from build123d import *

# Parameters (mm, degrees)
SKETCH1_W           = 101.6
SKETCH1_H           = 53.34
BOSS_EXTRUDE1_DEPTH = 1.524
SKETCH2_W           = 19.05
SKETCH2_H           = 19.05
BOSS_EXTRUDE2_DEPTH = 1.016
SKETCH3_W           = 14.918140665
SKETCH3_H           = 9.726042688
BOSS_EXTRUDE3_DEPTH = 12.7
SKETCH4_W           = 24.926999196
SKETCH4_H           = 1.692574019
SKETCH4_W_2         = 22.820903589
SKETCH4_H_2         = 2.077249933
SKETCH4_W_3         = 16.079453185
SKETCH4_H_3         = 2.769666577
SKETCH4_W_4         = 2.00031475
SKETCH4_H_4         = 36.313406236
SKETCH4_W_5         = 30.004721254
SKETCH4_W_6         = 23.772971456
SKETCH4_H_5         = 2.615796212
BOSS_EXTRUDE4_DEPTH = 9.525


with BuildPart() as part:
    # Sketch1 → Boss-Extrude1 (new body)
    with BuildSketch(Plane(origin=(0, 0, 0), x_dir=(1, 0, 0), z_dir=(0, 1, 0))):
        Rectangle(SKETCH1_W, SKETCH1_H)
    extrude(amount=BOSS_EXTRUDE1_DEPTH)

    # Sketch2 → Boss-Extrude2 (add)
    with BuildSketch(Plane(origin=(0, 1.524, 0), x_dir=(1, 0, 0), z_dir=(0, 1, 0))):
        Rectangle(SKETCH2_W, SKETCH2_H)
    extrude(amount=BOSS_EXTRUDE2_DEPTH)

    # Sketch3 → Boss-Extrude3 (add)
    with BuildSketch(Plane(origin=(0, 1.524, 0), x_dir=(1, 0, 0), z_dir=(0, 1, 0))):
        with Locations((-48.63021344, -18.537983619)):
            Rectangle(SKETCH3_W, SKETCH3_H)
    extrude(amount=BOSS_EXTRUDE3_DEPTH)

    # Sketch4 → Boss-Extrude4 (add)
    with BuildSketch(Plane(origin=(0, 1.524, 0), x_dir=(1, 0, 0), z_dir=(0, 1, 0))):
        with Locations((-20.570539456, 24.619258466)):
            Rectangle(SKETCH4_W, SKETCH4_H)
        with Locations((11.410451795, 23.580633498)):
            Rectangle(SKETCH4_W_2, SKETCH4_H_2)
        with Locations((40.092852107, 23.234425177)):
            Rectangle(SKETCH4_W_3, SKETCH4_H_3)
        with Locations((48.517254612, 0.538546279)):
            Rectangle(SKETCH4_W_4, SKETCH4_H_4)
        with Locations((33.514893985, -24.811596423)):
            Rectangle(SKETCH4_W_5, SKETCH4_H_2)
        with Locations((-2.683109477, -24.542323283)):
            Rectangle(SKETCH4_W_6, SKETCH4_H_5)
    extrude(amount=BOSS_EXTRUDE4_DEPTH)


solid = part.part
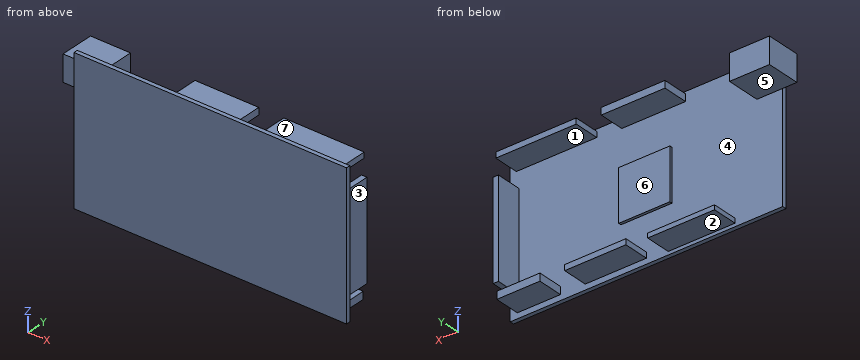
Geometry: final body of the model. Coordinates: model frame, mm. Face numbers are marked on the shaded views. A direction names the side the tool comes from. Coordinates: 2 decimals unless noted, no trailing zeros. Write each loop counter-clockwise with the first axis right and the second up, starting at its lowest first coordinate (ties: lowest second). Pieces come first, ordered by that corner, then holes. Notation, with made-up numbers: (70, 55) - (127, 55) arc R31 cw to (127, 92) - close; hole circle Ø10 at (9, 45). An arc over 180 degrees is marked (long way). Return JSON: item names as keys, results as strings.
Item 1: Reachability of the marked faces 5, 6 and 7 from +Z, -Z, +X, -X, +Y, -Y: full face, straight path, thin tool, end or side. Return the list, or none.
Completed:
{"face 5": "-Z, -X, +Y", "face 6": "-X, +Y", "face 7": "+Z, +X, -X, +Y"}
Item 2: Section query C-C (z = 4.5). Output: boundary loops of the cut face in (x, y) (3 decimals), and give its area (3 significant figures).
Completed:
{"outline": "(-50.8, 0) - (50.8, 0) - (50.8, 1.524) - (49.517, 1.524) - (49.517, 11.049) - (47.517, 11.049) - (47.517, 1.524) - (9.525, 1.524) - (9.525, 2.54) - (-9.525, 2.54) - (-9.525, 1.524) - (-50.8, 1.524) - close", "area": "193 mm2"}
Item 3: Section query D-D (x = -49). Output: boundary loops of the cut face in (y, z).
Completed:
{"outline": "(0, -26.67) - (1.52, -26.67) - (1.52, 13.67) - (14.22, 13.67) - (14.22, 23.4) - (1.52, 23.4) - (1.52, 26.67) - (0, 26.67) - close"}
Item 4: Pull-direction query (Z, two-part tool) for the marked faces 1, 2, 3 and 4; classes: +Z half, -Z half, draft (parallel to the pull), parting line (faces both ways), or undercut.
Completed:
{"face 1": "undercut", "face 2": "-Z half", "face 3": "draft", "face 4": "undercut"}
Item 5: Section query A-A (y = 7). Output: boundary loops of the cut face in (x, z), and give its area (3 significant figures).
Completed:
{"outline": "(-56.09, 13.67) - (-41.17, 13.67) - (-41.17, 23.4) - (-56.09, 23.4) - close; (-33.03, -25.47) - (-8.11, -25.47) - (-8.11, -23.77) - (-33.03, -23.77) - close; (-14.57, 23.23) - (9.2, 23.23) - (9.2, 25.85) - (-14.57, 25.85) - close; (0, -24.62) - (22.82, -24.62) - (22.82, -22.54) - (0, -22.54) - close; (18.51, 23.77) - (48.52, 23.77) - (48.52, 25.85) - (18.51, 25.85) - close; (32.05, -24.62) - (48.13, -24.62) - (48.13, -21.85) - (32.05, -21.85) - close; (47.52, -18.7) - (49.52, -18.7) - (49.52, 17.62) - (47.52, 17.62) - close", "area": "476 mm2"}
Item 6: Section query B-B (x = -11). Output: boundary loops of the cut face in (y, z), and give its area (3 significant figures).
Completed:
{"outline": "(0, -26.67) - (1.52, -26.67) - (1.52, -25.47) - (11.05, -25.47) - (11.05, -23.77) - (1.52, -23.77) - (1.52, 23.23) - (11.05, 23.23) - (11.05, 25.85) - (1.52, 25.85) - (1.52, 26.67) - (0, 26.67) - close", "area": "122 mm2"}
Item 7: Pin query (flat end, axial travel): pin 1 Ø4 at (x, z) = (-25, 17.5) entering from -Y; pin 2 Ø5 at (x, y) = (-3.5, 7.5) entering from -Z; pin 3 Ø3 at (y, z) = (6, -23) entering from -X; pin 4 Ø0.8 at (x, z) = (41.5, -23) entering from +Y. Return the tip coordinate at first contact, or that it passes through.
Completed:
{"pin 1": "stops at y = 0", "pin 2": "stops at z = 23.23", "pin 3": "stops at x = -33.03", "pin 4": "stops at y = 11.05"}
Item 8: Line query: L1, parallel to Z at x = 22, y = 2.5; L2, parallel to Z at x = -12, y = 5.25; L3, parallel to X at y = 3.5, z = 14. Output: solid intervals per line, ascending.
Completed:
{"L1": "z = -24.62 to -22.54, 23.77 to 25.85", "L2": "z = -25.47 to -23.77, 23.23 to 25.85", "L3": "x = -56.09 to -41.17, 47.52 to 49.52"}
